Design review of the part shown in the three views and the two pictorial views. Dimensions are in mm from the part's minimum x, y and z. Coordinates: 2 decimals unless noted, no trailing zeros. Loops run counter-clockwise (first coordinate to the right, second up) from the corner with the lowest first, then second, coordinate; pieces in that order, holes last. Notation, with made-up numbers: (19.25, -23.5) - (76.25, -23.5) arc R8 ccw to (76.25, -10.5) - close; hole circle Ø7 at (9, 88.25). An arc over 180 degrees is marked (long way). One line per item, written item: value. Start each with the question number.
1. To check wall thickness, follow line 1 (X direction, y = 3, z = 0.5) (1 decimal); line 2 (X direction, y = 3.5, z = 1.55) (1 decimal); line 3 (Y direction, x = 14.5, z = 0.55) (1 decimal). State the ranges of each line that lie inside material, in increasing order. Write a range as from..to.
2. Take a section at D-D, the plane x = 17. State the section outline as (y, z) points.
3. Take a section at C-C, the plane z = 1.15. Count the separate pieces of the cut face and the enclosed holes in it.
4. Take a section at B-B, the plane x = 36. State the section outline as (y, z) points (1 decimal).
5. Take a section at A-A, the plane y = 21. State the section outline as (x, z) points.
6. Insertion check: pin 1 (22.5 mm diameter, centred on x = 21.2, y = 19.2, fed in from -Z). The pin has a flat end and moves straight along its axis. Give the tip position at first contact, or say it passes through.
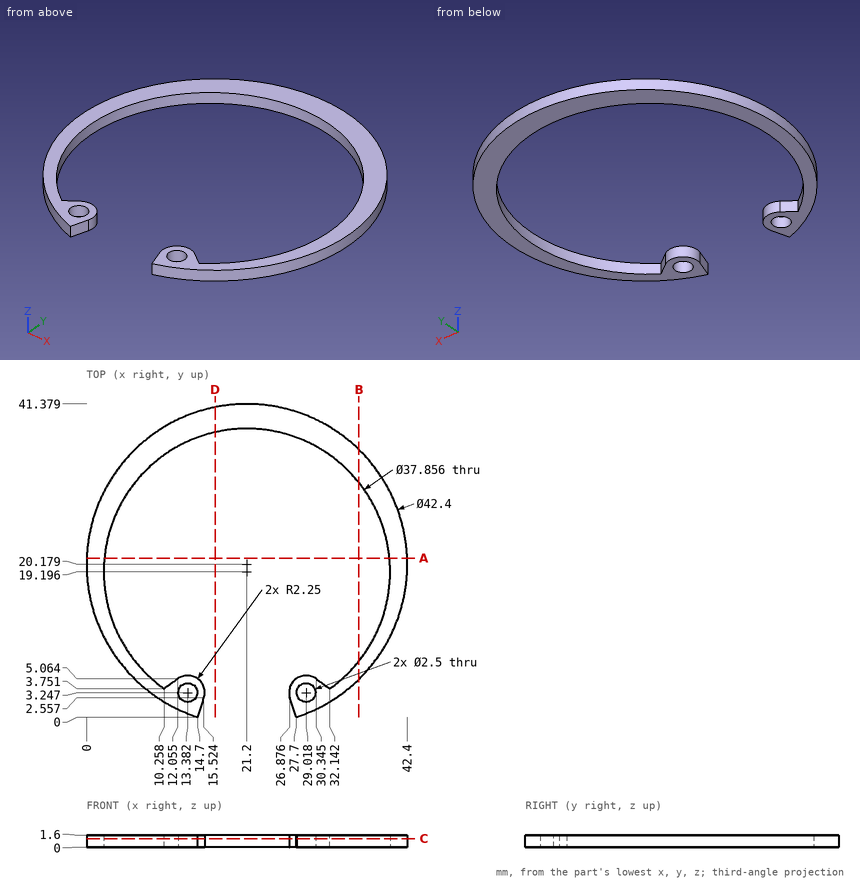
Solutions:
1. line 1: 8.8..12.2, 14.6..15.6, 26.8..27.8, 30.2..33.6
1. line 2: 8.1..12.2, 14.6..15.6, 26.8..27.8, 30.2..34.3
1. line 3: 0.1..2.7, 3.8..5.2, 36.9..40.3
2. outline: (37.65, 0) - (40.96, 0) - (40.96, 1.6) - (37.65, 1.6) - close
3. separate pieces: 1
3. enclosed holes: 2
4. outline: (5, 0) - (7.4, 0) - (7.4, 1.6) - (5, 1.6) - close; (31, 0) - (35.4, 0) - (35.4, 1.6) - (31, 1.6) - close
5. outline: (0.02, 0) - (2.36, 0) - (2.36, 1.6) - (0.02, 1.6) - close; (40.04, 0) - (42.38, 0) - (42.38, 1.6) - (40.04, 1.6) - close
6. pin 1: through
